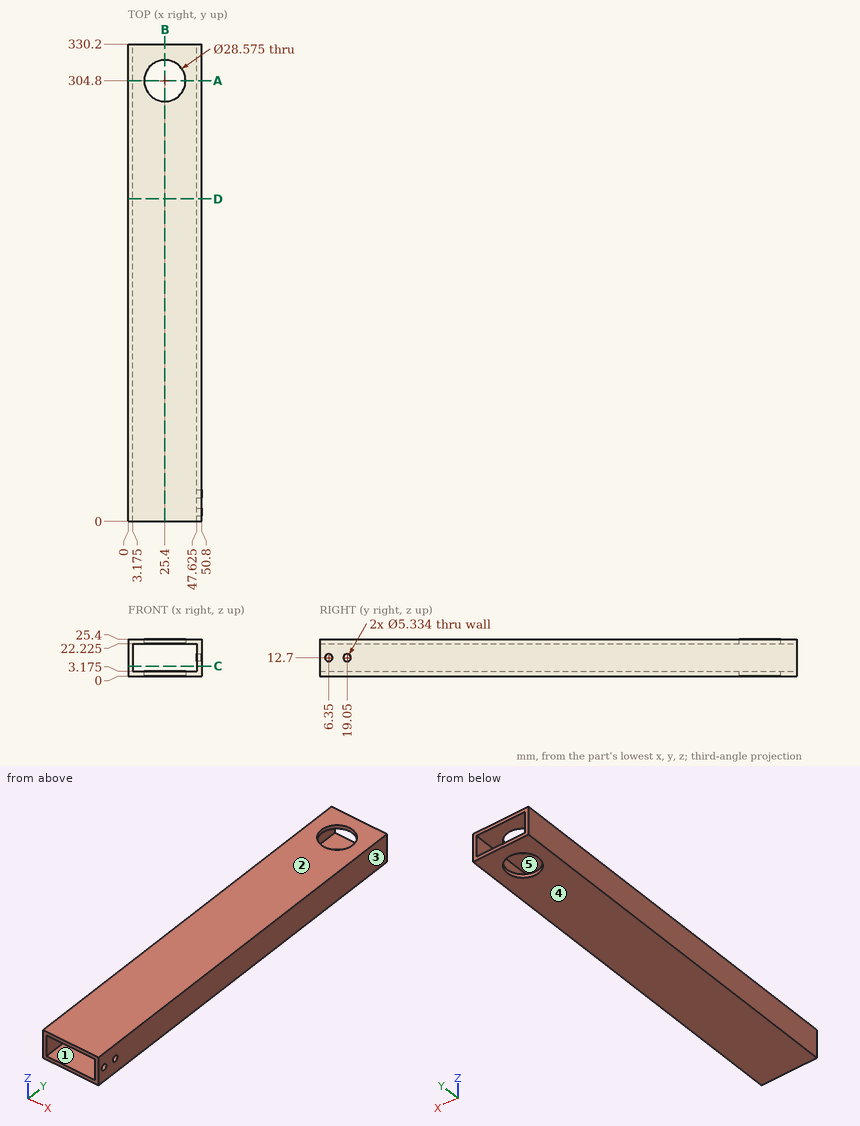
Source: three-view drawing plus pictorial views. Frame: mm from the lowest corner of the part. A direction names the side the tool comes from. Coordinates: 2 decimals unless noted, no trailing zeros. Order: outer loops, then holes, each group sorted by start corner. A loop starts at its lowest first (then second) coordinate and runs counter-clockwise, first axis right, second up. Notation, with made-up numbers: M -38,54 L -16,54 A12 ccw -16,69 Z; hole C -27,-5 d6. An arc over 180 degrees is marked long. Answer in a Markdown table with one row per item.
(1) Section query A-A, the plane y = 304.8. Output: boundary loops of the cut face in (x, z) (1 decimal), plus the area to 3 significant figures.
Numbers:
| item | result |
|---|---|
| outline | M 0,0 L 11.1,0 L 11.1,3.2 L 3.2,3.2 L 3.2,22.2 L 11.1,22.2 L 11.1,25.4 L 0,25.4 Z; M 39.7,0 L 50.8,0 L 50.8,25.4 L 39.7,25.4 L 39.7,22.2 L 47.6,22.2 L 47.6,3.2 L 39.7,3.2 Z |
| area | 262 mm^2 |
(2) Contact query for a flat-ended pin moving along its axis: pin 1 Ø5 at (y, z) = (6.35, 12.7) entering from +X (3 decimals). Output: stop coordinate, or through.
Numbers:
| item | result |
|---|---|
| pin 1 | stops at x = 3.175 |
(3) Section query D-D, the plane y = 223. Output: boundary loops of the cut face in (x, z) (3 decimals), plus the area to 3 significant figures.
Numbers:
| item | result |
|---|---|
| outline | M 0,0 L 50.8,0 L 50.8,25.4 L 0,25.4 Z; hole M 3.175,3.175 L 47.625,3.175 L 47.625,22.225 L 3.175,22.225 Z |
| area | 444 mm^2 |
(4) Section query C-C, the plane z = 6.75. Output: boundary loops of the cut face in (x, y) (3 decimals).
Numbers:
| item | result |
|---|---|
| outline | M 0,0 L 3.175,0 L 3.175,330.2 L 0,330.2 Z; M 47.625,0 L 50.8,0 L 50.8,330.2 L 47.625,330.2 Z |
(5) Access query for the marked faces 4 and 5. Directions: +Z, -Z, +X, -X, +Y, -Y. A direction counts if a zero-diameter tool reaches every point of the face in a straight line with its end or side. Return the directions, or none.
Numbers:
| item | result |
|---|---|
| face 4 | -Z, +X, -X, +Y, -Y |
| face 5 | +Y, -Y |
(6) Material intervals for line 1 (Y direction, x = 48.95, z = 12.7); line 2 (Z direction, x = 11.5, y = 16) (3 decimals); line 3 (X direction, y = 296, z = 13.5) (3 decimals), sorted ascending. Write a range as [from, to].
Numbers:
| item | result |
|---|---|
| line 1 | y = [0, 3.68], [9.02, 16.38], [21.72, 330.2] |
| line 2 | z = [0, 3.175], [22.225, 25.4] |
| line 3 | x = [0, 3.175], [47.625, 50.8] |
(7) Section query B-B, the plane x = 25.4. Output: boundary loops of the cut face in (y, z) (1 decimal), plus the area to 3 significant figures.
Numbers:
| item | result |
|---|---|
| outline | M 0,0 L 290.5,0 L 290.5,3.2 L 0,3.2 Z; M 0,22.2 L 290.5,22.2 L 290.5,25.4 L 0,25.4 Z; M 319.1,0 L 330.2,0 L 330.2,3.2 L 319.1,3.2 Z; M 319.1,22.2 L 330.2,22.2 L 330.2,25.4 L 319.1,25.4 Z |
| area | 1,920 mm^2 |
(8) Draft query along Z for the marked faces 1, 2 and 3. Return one class per face: pulls with the +Z half, pulls with the -Z half, needs draft (parallel to the pull), parting line crosses it, or undercut.
Numbers:
| item | result |
|---|---|
| face 1 | undercut |
| face 2 | pulls with the +Z half |
| face 3 | needs draft |
